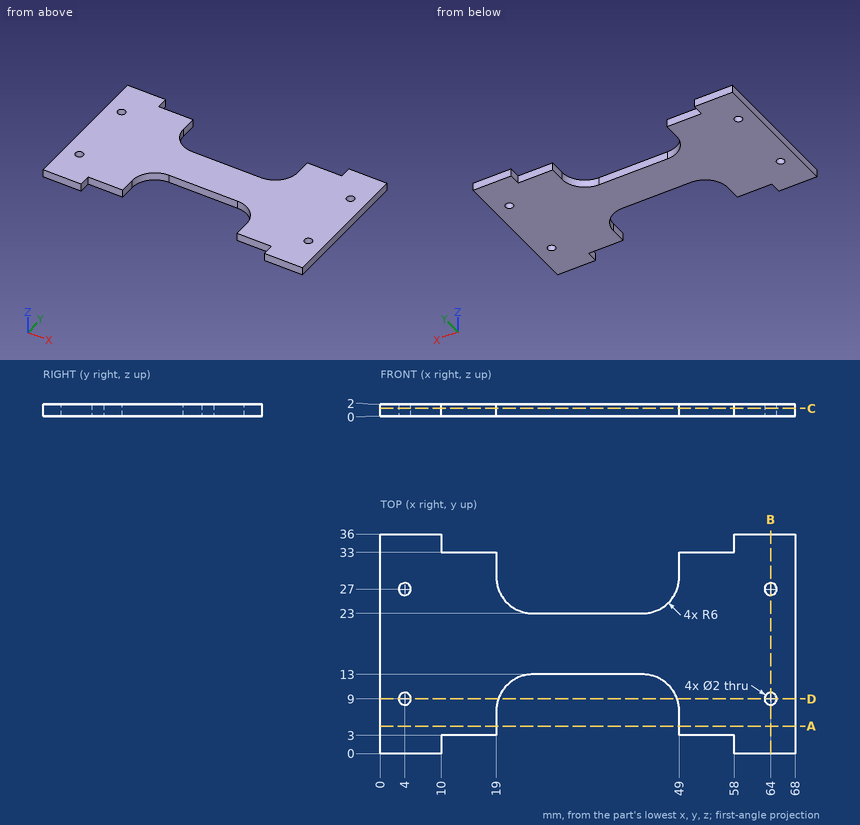
Geometry check sheet. Reference: drawing and pictorial views, mm from the part's lowest x, y, z. Give positions to 0.01 mm unless a question says otherwise; leave off trailing zeros. Order: outer loops, then holes, each group sorted by start corner. A loop starts at its lowest first (then second) coordinate and runs counter-clockwise, first axis right, second up. Notation, with made-up numbers: M 79,83.25 L 102,83.25 A23 ccw 102,121.25 Z; hole C 17.5,-10.5 d2. An arc over 180 degrees is marked long. Answer in a Markdown table with one row per item. Add a question column.
Q1. Sectioned sample at C-C, the plane z = 1.3. Record the boundary of the cut face in (x, y), and give its area (3 significant figures).
Q2. Sectioned sample at A-A, the plane y = 4.5. Record the boundary of the cut face in (x, z), and give its area (3 significant figures).
Q3. Thickness scan on L1, parallel to Y at x = 64, z = 1.15; L2, parallel to X at y = 34.5, z = 0.4; L3, parallel to X at y = 3.5, z = 0.45. Record the ranges inside material, lowest first.
Q4. Gauge pin test, flat ends, axial feed: pin 1 Ø4 at (x, y) = (38.5, 13.5) entering from -Z; pin 2 Ø1 at (x, z) = (15.5, 0.5) entering from -Y; pin 3 Ø0.6 at (x, z) = (52, 0.5) entering from +Y; pin 4 Ø1 at (x, z) = (35.5, 1) entering from -Y. Record the tip position at first contact, or that the pin passes through.
Q5. Sectioned sample at B-B, the plane x = 64. Record the boundary of the cut face in (y, z).
Q6. Sectioned sample at D-D, the plane y = 9. Record the boundary of the cut face in (x, z).
Verdict:
| question | item | result |
|---|---|---|
| 1 | outline | M 0,0 L 10,0 L 10,3 L 19,3 L 19,7 A6 cw 25,13 L 43,13 A6 cw 49,7 L 49,3 L 58,3 L 58,0 L 68,0 L 68,36 L 58,36 L 58,33 L 49,33 L 49,29 A6 cw 43,23 L 25,23 A6 cw 19,29 L 19,33 L 10,33 L 10,36 L 0,36 Z; hole C 4,9 d2; hole C 4,27 d2; hole C 64,9 d2; hole C 64,27 d2 |
| 1 | area | 1,580 mm² |
| 2 | outline | M 0,0 L 19,0 L 19,2 L 0,2 Z; M 49,0 L 68,0 L 68,2 L 49,2 Z |
| 2 | area | 76.0 mm² |
| 3 | L1 | 0 to 8, 10 to 26, 28 to 36 |
| 3 | L2 | 0 to 10, 58 to 68 |
| 3 | L3 | 0 to 19, 49 to 68 |
| 4 | pin 1 | z = 0 |
| 4 | pin 2 | y = 3 |
| 4 | pin 3 | y = 33 |
| 4 | pin 4 | y = 13 |
| 5 | outline | M 0,0 L 8,0 L 8,2 L 0,2 Z; M 10,0 L 26,0 L 26,2 L 10,2 Z; M 28,0 L 36,0 L 36,2 L 28,2 Z |
| 6 | outline | M 0,0 L 3,0 L 3,2 L 0,2 Z; M 5,0 L 19.34,0 L 19.34,2 L 5,2 Z; M 48.66,0 L 63,0 L 63,2 L 48.66,2 Z; M 65,0 L 68,0 L 68,2 L 65,2 Z |
